from build123d import *

# Parameters (mm, degrees)
SKETCH1_R            = 62.5
BOSS_EXTRUDE8_DEPTH  = 35
BOSS_EXTRUDE9_REACH  = 192.245
SKETCH2_W            = 15
SKETCH2_H            = 35
SKETCH10_W           = 35
SKETCH10_H           = 15
BOSS_EXTRUDE12_DEPTH = 40
SKETCH6_W            = 35
SKETCH6_H            = 15
BOSS_EXTRUDE10_DEPTH = 40
SKETCH12_W           = 42.229373335
SKETCH12_H           = 20
SKETCH12_W_2         = 40
SKETCH12_H_2         = 15
SKETCH12_W_3         = 39.995847529
BOSS_EXTRUDE13_DEPTH = 97.5
SKETCH13_W           = 20
SKETCH13_H           = 5
SKETCH13_W_2         = 25.5
SKETCH13_H_2         = 5.5
CUT_EXTRUDE1_DEPTH   = 20
SKETCH14_W           = 20
SKETCH14_H           = 5
SKETCH14_W_2         = 25.5
SKETCH14_H_2         = 5.5
BOSS_EXTRUDE14_DEPTH = 20


with BuildPart() as part:
    # Sketch1 → Boss-Extrude8 (new body)
    with BuildSketch(Plane.XY):
        with BuildLine():
            Line((127.600917431, -117.745016448), (72.5, 0))
            ThreePointArc((72.5, 0), (0, 72.5), (-72.5, 0))
            Line((-72.5, 0), (-127.600917431, -117.745016448))
            Line((-127.600917431, -117.745016448), (-167.600917431, -117.745016448))
            Line((-167.600917431, -117.745016448), (-167.600917431, -137.745016448))
            Line((-167.600917431, -137.745016448), (167.600917431, -137.745016448))
            Line((167.600917431, -137.745016448), (167.600917431, -117.745016448))
            Line((167.600917431, -117.745016448), (127.600917431, -117.745016448))
        make_face()
        with BuildLine():
            ThreePointArc((-67.21559633, -27.171926873), (0, -72.5), (67.21559633, -27.171926873))
            Line((67.21559633, -27.171926873), (101.417450928, -100.25778678))
            Line((101.417450928, -100.25778678), (88.408256881, -117.745016448))
            Line((88.408256881, -117.745016448), (-88.408256881, -117.745016448))
            Line((-88.408256881, -117.745016448), (-101.417450928, -100.25778678))
            Line((-101.417450928, -100.25778678), (-67.21559633, -27.171926873))
        make_face(mode=Mode.SUBTRACT)
        Circle(SKETCH1_R, mode=Mode.SUBTRACT)
    extrude(amount=BOSS_EXTRUDE8_DEPTH)

    # Sketch2 → Boss-Extrude9 (add, up to next)
    with BuildSketch(Plane(origin=(0, -117.745016448, 0), x_dir=(1, 0, 0), z_dir=(0, 1, 0)), mode=Mode.PRIVATE) as boss_extrude9_sk1:
        with Locations((0.093911399, -17.5)):
            Rectangle(SKETCH2_W, SKETCH2_H)
    boss_extrude9_tool1 = extrude(boss_extrude9_sk1.sketch, amount=BOSS_EXTRUDE9_REACH, mode=Mode.PRIVATE) - part.part
    add(boss_extrude9_tool1.solids().sort_by_distance((0.093911, -117.745016, 17.5))[0])

    # Sketch10 → Boss-Extrude12 (add)
    with BuildSketch(Plane(origin=(-72.5, 0, 0), x_dir=(0, 0, -1), z_dir=(1, 0, 0))):
        with Locations((-17.5, -7.5)):
            Rectangle(SKETCH10_W, SKETCH10_H)
    extrude(amount=-BOSS_EXTRUDE12_DEPTH)

    # Sketch6 → Boss-Extrude10 (add)
    with BuildSketch(Plane(origin=(72.5, 0, 0), x_dir=(0, 0, -1), z_dir=(1, 0, 0))):
        with Locations((-17.5, -7.5)):
            Rectangle(SKETCH6_W, SKETCH6_H)
    extrude(amount=BOSS_EXTRUDE10_DEPTH)

    # Sketch12 → Boss-Extrude13 (add)
    with BuildSketch(Plane(origin=(0, 0, 0), x_dir=(-1, 0, 0), z_dir=(0, 0, -1))):
        with Locations((-146.486230764, -127.745016448)):
            Rectangle(SKETCH12_W, SKETCH12_H)
        with Locations((147.600917431, -127.745016448)):
            Rectangle(SKETCH12_W_2, SKETCH12_H)
        with Locations((-92.5, -7.5)):
            Rectangle(SKETCH12_W_2, SKETCH12_H_2)
        with Locations((92.502076235, -7.5)):
            Rectangle(SKETCH12_W_3, SKETCH12_H_2)
    extrude(amount=BOSS_EXTRUDE13_DEPTH)

    # Sketch13 → Cut-Extrude1 (cut)
    with BuildSketch(Plane.XY.offset(35)):
        with Locations((-92.5, -12.5)):
            Rectangle(SKETCH13_W, SKETCH13_H)
        with Locations((-147.600917431, -134.995016448)):
            Rectangle(SKETCH13_W_2, SKETCH13_H_2)
        with Locations((-92.5, -2.5)):
            Rectangle(SKETCH13_W, SKETCH13_H)
        with Locations((92.5, -2.5)):
            Rectangle(SKETCH13_W, SKETCH13_H)
        with Locations((92.5, -12.5)):
            Rectangle(SKETCH13_W, SKETCH13_H)
        with Locations((147.600917431, -120.495016448)):
            Rectangle(SKETCH13_W_2, SKETCH13_H_2)
        with Locations((147.600917431, -134.995016448)):
            Rectangle(SKETCH13_W_2, SKETCH13_H_2)
        with Locations((-147.600917431, -120.495016448)):
            Rectangle(SKETCH13_W_2, SKETCH13_H_2)
    extrude(amount=-CUT_EXTRUDE1_DEPTH, mode=Mode.SUBTRACT)

    # Sketch14 → Boss-Extrude14 (add)
    with BuildSketch(Plane(origin=(0, 0, -97.5), x_dir=(-1, 0, 0), z_dir=(0, 0, -1))):
        with Locations((-92.5, -2.5)):
            Rectangle(SKETCH14_W, SKETCH14_H)
        with Locations((-92.5, -12.5)):
            Rectangle(SKETCH14_W, SKETCH14_H)
        with Locations((92.5, -2.5)):
            Rectangle(SKETCH14_W, SKETCH14_H)
        with Locations((92.5, -12.5)):
            Rectangle(SKETCH14_W, SKETCH14_H)
        with Locations((147.600917431, -120.495016448)):
            Rectangle(SKETCH14_W_2, SKETCH14_H_2)
        with Locations((147.600917431, -134.995016448)):
            Rectangle(SKETCH14_W_2, SKETCH14_H_2)
        with Locations((-147.600917431, -120.495016448)):
            Rectangle(SKETCH14_W_2, SKETCH14_H_2)
        with Locations((-147.600917431, -134.995016448)):
            Rectangle(SKETCH14_W_2, SKETCH14_H_2)
    extrude(amount=BOSS_EXTRUDE14_DEPTH)


solid = part.part
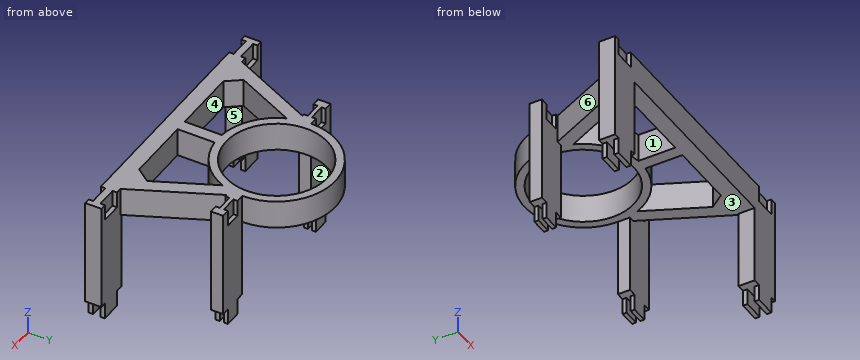
Verification items for the finished model (mm, model axes). Face numbers are marked on the shaded views. A direction names the side the tool comes from. Coordinates: 2 decimals unless noted, no trailing zeros. Write each loop counter-clockwise with the first axis right and the second up, starting at its lowest first coordinate (ties: lowest second). Pieces come first, ordered by that corner, then holes. Notation, with made-up numbers: M 85,60 L 96,60 A15 cw 96,68 Z; hole C 5,-23 d4. An arc over 180 degrees is marked long. Use CSV: the item, a comma, the result in double quotes.
Q1. Mould release check, pull along Y, two halves, no side actions. Record for the marked faces 1, 2 and 3: pulls with the +Y half, pulls with the -Y half, needs draft (parallel to the pull), parting line crosses it, or undercut.
Computed values:
face 1,"undercut"
face 2,"pulls with the +Y half"
face 3,"needs draft"
Q2. Go/stop test with flat-tipped pins: P1, Ø2.5, axis at x = 88, y = -1.5, coming from the +Z side; P2, Ø10, axis at x = -74, z = -70, coming from the -Y side; P3, Ø1.5, axis at y = -40, z = 3, coming from the +X side. Record where each tip stops, or that it passes through.
Computed values:
P1,"z = 15"
P2,"y = -15"
P3,"x = 91.57"
Q3. Section check A-A, the plane x = 0. Enter the section's corners in (y, z).
Computed values:
outline,"M -137.75,0 L -62.5,0 L -62.5,35 L -137.75,35 Z; M 62.5,0 L 72.5,0 L 72.5,35 L 62.5,35 Z"
Q4. Section check B-B, the plane z = -89. Enter the section's corners in (x, y).
Computed values:
outline,"M -167.6,-137.75 L -127.6,-137.75 L -127.6,-117.75 L -167.6,-117.75 Z; M -112.5,-15 L -72.5,-15 L -72.5,0 L -112.5,0 Z; M 72.5,-15 L 112.5,-15 L 112.5,0 L 72.5,0 Z; M 125.37,-137.75 L 167.6,-137.75 L 167.6,-117.75 L 125.37,-117.75 Z"
Q5. Thickness scan on line 1 along Y through (x, z) = (0, 27); line 2 along X through (y, z) = (-53.5, 5.5); line 3 along Y through (x, z) = (79, -56.5). Record the ranges inside material, lowest first. Write a range as [from, to].
Computed values:
line 1,"[-137.75, -62.5], [62.5, 72.5]"
line 2,"[-97.54, -79.54], [-48.93, -32.31], [32.31, 48.93], [79.54, 97.54]"
line 3,"[-15, 0]"
Q6. Section check C-C, the plane y = 7. Enter the section's corners in (x, z), and give its area (3 significant figures).
Computed values:
outline,"M -72.16,0 L -62.11,0 L -62.11,35 L -72.16,35 Z; M 62.11,0 L 72.16,0 L 72.16,35 L 62.11,35 Z"
area,"704 mm²"
Q7. Set-up check for the marked faces 4, 5 and 6: record each of +Z, -Z, +X, -X, +Y, -Y from which the full face is reachable in a straight line by a thin tool's end or side.
Computed values:
face 4,"+Z, -Z"
face 5,"-Z, +Y, -Y"
face 6,"+Z, -Z, -X"
